Input: dimensioned drawing with shaded views. Units: mm. Origin: part minimum x, y, z. A direction names the side the tool comes from. Coordinates: 2 decimals unless noted, no trailing zeros. Order: outer loops, then holes, each group sorted by start corner. A loop starts at its lowest first (then second) coordinate and runs counter-clockwise, first axis right, second up.
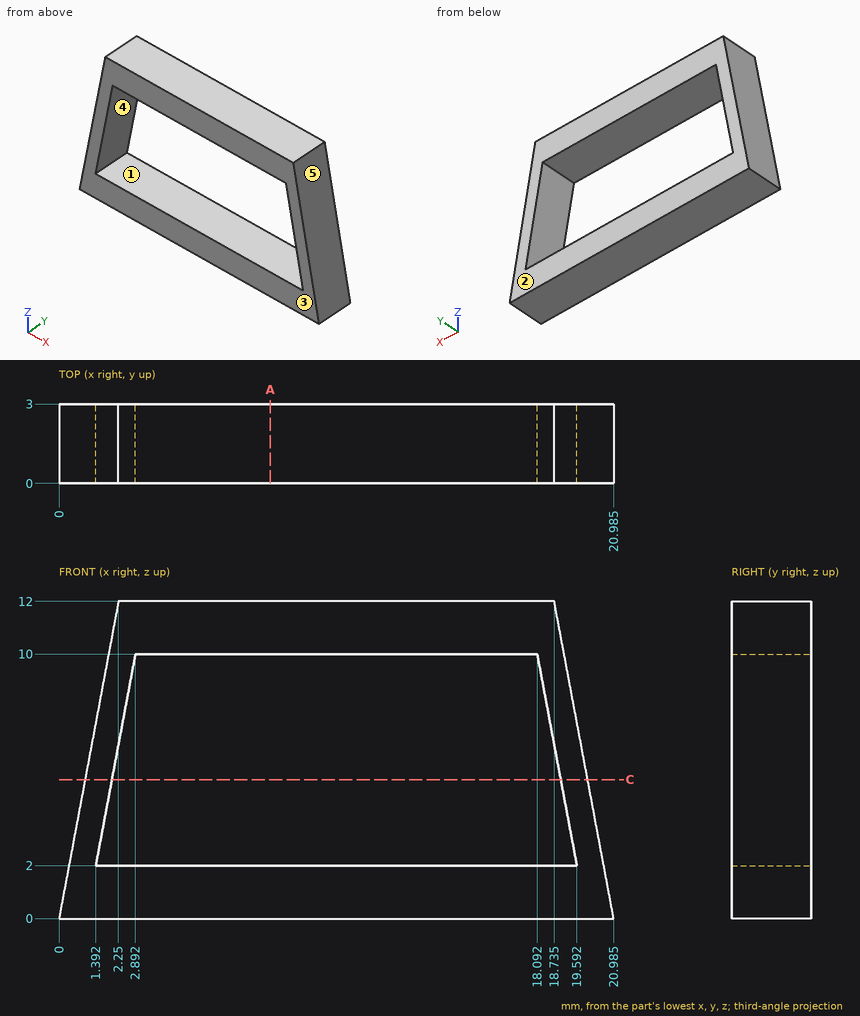
1. Ray query, line 1 (Z direction, x = 11.75, y = 2.5); line 2 (X direction, y = 1.7, z = 4.5); line 3 (X direction, y = 2.3, z = 9.75) (1 decimal). Return the intervals inside material, ascending.
Findings:
line 1: z = 0 to 2, 10 to 12
line 2: x = 0.84 to 1.86, 19.12 to 20.14
line 3: x = 1.8 to 2.8, 18.1 to 19.2
2. Section query C-C on z = 5.25. Return loops of the section in (x, y) (1 decimal).
Findings:
outline: (1, 0) - (2, 0) - (2, 3) - (1, 3) - close; (19, 0) - (20, 0) - (20, 3) - (19, 3) - close
3. Section query A-A on x = 8. Return loops of the section in (y, z), plus the area to 3 significant figures.
Findings:
outline: (0, 0) - (3, 0) - (3, 2) - (0, 2) - close; (0, 10) - (3, 10) - (3, 12) - (0, 12) - close
area: 12.0 mm2
4. Draft query along X for the marked faces 3, 4 and 5. Return one class per face: released by +X, released by -X, zero draft, split by the parting line, or undercut.
Findings:
face 3: zero draft
face 4: undercut
face 5: released by +X
5. Access query for the marked faces 1 and 2. Directions: +Z, -Z, +X, -X, +Y, -Y. A direction counts if a zero-diameter tool reaches every point of the face in a straight line with its end or side. Return the directions, or none.
Findings:
face 1: +Y, -Y
face 2: +Z, -Z, +X, -X, +Y
